from build123d import *

# Parameters (mm, degrees)
BOSS_EXTRU_1_DEPTH           = 125
ESQUISSE2_R                  = 2.45
BOSS_EXTRU_2_DEPTH           = 8
CONG_1_R                     = 0.75
COQUE1_START                 = -122.5
COQUE1_DEPTH                 = 245
ENL_V_MAT_EXTRU_1_DEPTH      = 162.382066666
ESQUISSE4_R                  = 3.25
ESQUISSE4_R_2                = 1.65
BOSS_EXTRU_3_DEPTH           = 6
R_P_TITION_CIRCULAIRE1_COUNT = 2
BOSS_EXTRU_4_DEPTH           = 1.8


# Read off the part's stored shape, not the designer's step: Coque1
with BuildPart() as part:
    # Esquisse1 → Boss.-Extru.1 (new body)
    with BuildSketch(Plane(origin=(0, 0, 0), x_dir=(0, 0, -1), z_dir=(1, 0, 0))):
        Polygon((5, 15.857974012), (0, 0), (-5, 15.857974012), (-5, 90.857974012), (5, 90.857974012), align=None)
    boss_extru_1 = extrude(amount=BOSS_EXTRU_1_DEPTH)

    # Esquisse2 → Boss.-Extru.2 (add)
    with BuildSketch(Plane.ZY.offset(-125)):
        with Locations((0, 11.639283332)):
            Circle(ESQUISSE2_R)
    boss_extru_2 = extrude(amount=-BOSS_EXTRU_2_DEPTH)

    # Symétrie1: Boss.-Extru.1, Boss.-Extru.2 across plane
    add(boss_extru_1.mirror(Plane(origin=(0, 0, 0), x_dir=(0, 0, 1), z_dir=(1, 0, 0))))
    add(boss_extru_2.mirror(Plane(origin=(0, 0, 0), x_dir=(0, 0, 1), z_dir=(1, 0, 0))))

    # Congé1
    cong_1_edges = [part.edges().sort_by_distance(p)[0] for p in [
        (0, 0, 0),
    ]]
    fillet(cong_1_edges, radius=CONG_1_R)

    # Coque1 outline → Coque1 (cut)
    with BuildSketch(Plane.YZ.offset(COQUE1_START)):
        Polygon((16.242760814, 2.5), (4.156886904, -1.310661406), (15.857974012, -5), (88.357974012, -5), (88.357974012, 2.5), align=None)
    extrude(amount=COQUE1_DEPTH, mode=Mode.SUBTRACT)

    # Esquisse3 → Enlèv. mat.-Extru.1 (cut, through all)
    with BuildSketch(Plane.XY.offset(5)):
        with BuildLine():
            Line((116.7, 19.857974012), (116.7, 24.857974012))
            ThreePointArc((116.7, 24.857974012), (114.560923955, 27.331783604), (111.804212881, 25.572259726))
            ThreePointArc((111.804212881, 25.572259726), (111.443512338, 25.056190286), (110.845898034, 24.857974012))
            Line((110.845898034, 24.857974012), (12.7, 24.857974012))
            ThreePointArc((12.7, 24.857974012), (11.992893219, 24.565080793), (11.7, 23.857974012))
            Line((11.7, 23.857974012), (11.7, 20.857974012))
            ThreePointArc((11.7, 20.857974012), (11.992893219, 20.150867231), (12.7, 19.857974012))
            Line((12.7, 19.857974012), (110.845898034, 19.857974012))
            ThreePointArc((110.845898034, 19.857974012), (111.443512338, 19.659757738), (111.804212881, 19.143688298))
            ThreePointArc((111.804212881, 19.143688298), (114.560923955, 17.38416442), (116.7, 19.857974012))
        make_face()
    enl_v_mat_extru_1 = extrude(amount=-ENL_V_MAT_EXTRU_1_DEPTH, mode=Mode.SUBTRACT)

    # Esquisse4 → Boss.-Extru.3 (add)
    with BuildSketch(Plane(origin=(0, 0, 2.5), x_dir=(-1, 0, 0), z_dir=(0, 0, -1))):
        with Locations(Location((0, 34.857974012, 0), (0, 0, 90))):
            Circle(ESQUISSE4_R)
        with Locations(Location((0, 34.857974012, 0), (0, 0, 90))):
            Circle(ESQUISSE4_R_2, mode=Mode.SUBTRACT)
    extrude(amount=BOSS_EXTRU_3_DEPTH)

    # Répétition circulaire1: Enlèv. mat.-Extru.1 ×2 about axis
    r_p_tition_circulaire1_axis = Axis((0, 34.857974012, 0), (0, 0, 1))
    for i in range(1, R_P_TITION_CIRCULAIRE1_COUNT):
        add(enl_v_mat_extru_1.rotate(r_p_tition_circulaire1_axis, i * 360 / R_P_TITION_CIRCULAIRE1_COUNT), mode=Mode.SUBTRACT)

    # Esquisse5 → Boss.-Extru.4 (add)
    with BuildSketch(Plane(origin=(0, 0, 2.5), x_dir=(-1, 0, 0), z_dir=(0, 0, -1))):
        with BuildLine():
            Line((-13.95, 39.857974012), (-13.95, 29.857974012))
            ThreePointArc((-13.95, 29.857974012), (-13.25, 29.157974012), (-12.55, 29.857974012))
            Line((-12.55, 29.857974012), (-12.55, 39.857974012))
            ThreePointArc((-12.55, 39.857974012), (-13.25, 40.557974012), (-13.95, 39.857974012))
        make_face()
        with BuildLine():
            Line((12.55, 39.857974012), (12.55, 29.857974012))
            ThreePointArc((12.55, 29.857974012), (13.25, 29.157974012), (13.95, 29.857974012))
            Line((13.95, 29.857974012), (13.95, 39.857974012))
            ThreePointArc((13.95, 39.857974012), (13.25, 40.557974012), (12.55, 39.857974012))
        make_face()
        with BuildLine():
            Line((-12.7, 26.257974012), (122.5, 26.257974012))
            ThreePointArc((122.5, 26.257974012), (123.2, 25.557974012), (122.5, 24.857974012))
            Line((122.5, 24.857974012), (-12.7, 24.857974012))
            Line((-12.7, 24.857974012), (-110.845898034, 24.857974012))
            ThreePointArc((-110.845898034, 24.857974012), (-111.545898034, 25.557974012), (-110.845898034, 26.257974012))
            Line((-110.845898034, 26.257974012), (-12.7, 26.257974012))
        make_face()
        with BuildLine():
            Line((-122.5, 15.857974012), (122.5, 15.857974012))
            ThreePointArc((122.5, 15.857974012), (123.2, 16.557974012), (122.5, 17.257974012))
            Line((122.5, 17.257974012), (-122.5, 17.257974012))
            ThreePointArc((-122.5, 17.257974012), (-123.2, 16.557974012), (-122.5, 15.857974012))
        make_face()
        with BuildLine():
            Line((12.7, 43.457974012), (-122.5, 43.457974012))
            ThreePointArc((-122.5, 43.457974012), (-123.2, 44.157974012), (-122.5, 44.857974012))
            Line((-122.5, 44.857974012), (12.7, 44.857974012))
            Line((12.7, 44.857974012), (110.845898034, 44.857974012))
            ThreePointArc((110.845898034, 44.857974012), (111.545898034, 44.157974012), (110.845898034, 43.457974012))
            Line((110.845898034, 43.457974012), (12.7, 43.457974012))
        make_face()
        with BuildLine():
            Line((-122.5, 52.457974012), (122.5, 52.457974012))
            ThreePointArc((122.5, 52.457974012), (123.2, 53.157974012), (122.5, 53.857974012))
            Line((122.5, 53.857974012), (-122.5, 53.857974012))
            ThreePointArc((-122.5, 53.857974012), (-123.2, 53.157974012), (-122.5, 52.457974012))
        make_face()
    extrude(amount=BOSS_EXTRU_4_DEPTH)


solid = part.part
Read the model definition and answer for the solid it produces. Units are mm, in the model's axes. A direction names the side the tool comes from. Round coordinates to 2 decimals unless told otherwise and drop trailing zeros. Write each loop counter-clockwise with the first axis right and the second up, starting at its lowest first coordinate (ties: lowest second). Pieces come first, ordered by that corner, then holes.
1. The part is cut by section B-B, the plane y = 65.5. Determine the outline of the cut face in (x, z).
2. Which of the six approach directions +Z, -Z, +X, -X, +Y, -Y give full straight-line access (tool end or side, diameter ignored) to faces 4 (the face through (128.94, 14.07, -0.32)), 5 (the face through (0.14, 31.61, -0.46)), 6 (the face through (2, 90.858, 0))?
3. The part is cut by section A-A, the plane x = 41. Determine the outline of the cut face in (y, z).
4. Straight lines are drawn through the part: L1, parallel to X at y = 82.5, z = -4.25; L2, parallel to X at y = 49, z = 4.5; L3, parallel to Z at x = -44.5, y = 84. For each, find the intervals that lie inside material, in ascending order.
5. Determine the mould class of faces 1 (the face through (-2, 88.358, -1)), 2 (the face through (-128.94, 14.07, -0.32)), 3 (the face through (-133, 12, 0)) for opening direction X: pulls with the +X half, pulls with the -X half, needs draft (parallel to the pull), parting line crosses it, or undercut.
6. Given pin 1 Ø1.5 at (x, y) = (13, 32.5) entering from -Z; pin 2 Ø0.9 at (y, z) = (34, 2) entering from +X; pin 3 Ø1.4 at (y, z) = (33, 1.5) entering from -X, each flat-ended and moving along its own axis, determine where each tip first touches the part or whether it passes through.
Values:
1. outline: (-125, -5) - (-122.5, -5) - (-122.5, 2.5) - (122.5, 2.5) - (122.5, -5) - (125, -5) - (125, 5) - (-125, 5) - close
2. face 4: +X
2. face 5: -Z
2. face 6: +Z, -Z, +X, -X, +Y
3. outline: (2.27, -0.72) - (4.16, -1.31) - (15.86, 2.38) - (15.86, 0.7) - (17.26, 0.7) - (17.26, 2.5) - (19.86, 2.5) - (19.86, 5) - (15.86, 5) - (2.27, 0.72) arc R0.75 ccw to start; (24.86, 0.7) - (26.26, 0.7) - (26.26, 2.5) - (43.46, 2.5) - (43.46, 0.7) - (44.86, 0.7) - (44.86, 2.5) - (52.46, 2.5) - (52.46, 0.7) - (53.86, 0.7) - (53.86, 2.5) - (88.36, 2.5) - (88.36, -5) - (90.86, -5) - (90.86, 5) - (24.86, 5) - close
4. L1: x = -125 to -122.5, 122.5 to 125
4. L2: x = -125 to -116.7, -11.71 to 125
4. L3: z = 2.5 to 5
5. face 1: undercut
5. face 2: needs draft
5. face 3: pulls with the -X half
6. pin 1: stops at z = 0.7
6. pin 2: stops at x = 125
6. pin 3: stops at x = -125
